```python
from build123d import *

# Parameters (mm, degrees)
SKETCH2_R           = 2.5
BOSS_EXTRUDE1_DEPTH = 5
SKETCH3_R           = 2.5
SKETCH3_R_2         = 0.5
BOSS_EXTRUDE2_DEPTH = 15.4


with BuildPart() as part:
    # Sketch2 → Boss-Extrude1 (new body)
    with BuildSketch(Plane.XY):
        with BuildLine():
            Line((-62, 4), (0, 4))
            ThreePointArc((0, 4), (1.530733729, 3.69551813), (2.828427125, 2.828427125))
            Line((2.828427125, 2.828427125), (17.67766953, -12.02081528))
            ThreePointArc((17.67766953, -12.02081528), (18.382077171, -16.725163117), (14.09037667, -18.776598105))
            Line((14.09037667, -18.776598105), (-62.758865735, -3.9273557))
            ThreePointArc((-62.758865735, -3.9273557), (-65.981797509, 0.381167417), (-62, 4))
        make_face()
        with Locations((-62, 0)):
            Circle(SKETCH2_R, mode=Mode.SUBTRACT)
        Circle(SKETCH2_R, mode=Mode.SUBTRACT)
    extrude(amount=BOSS_EXTRUDE1_DEPTH)

    # Sketch3 → Boss-Extrude2 (add)
    with BuildSketch(Plane(origin=(0, 0, 0), x_dir=(-1, 0, 0), z_dir=(0, 0, -1))):
        with Locations(Location((-14.849242405, -14.849242405, 0), (0, 0, 180))):
            Circle(SKETCH3_R)
        with Locations((-14.849242405, -14.849242405)):
            Circle(SKETCH3_R_2, mode=Mode.SUBTRACT)
    extrude(amount=BOSS_EXTRUDE2_DEPTH)


solid = part.part
```
Here's how the part is built. I have some questions about the finished solid (model axes, mm). A direction names the side the tool comes from. Coordinates: 2 decimals unless noted, no trailing zeros. Order: outer loops, then holes, each group sorted by start corner. A loop starts at its lowest first (then second) coordinate and runs counter-clockwise, first axis right, second up.
Item 1: If we section it at B-B, the plane y = -13.25: List the corners of the cut face in (x, z) for me, then the cut area to 3 significant figures.
Response values:
outline: (-14.51, 0) - (12.93, 0) - (12.93, -15.4) - (16.77, -15.4) - (16.77, 0) - (18.52, 0) - (18.52, 5) - (-14.51, 5) - close
area: 224 mm2
Item 2: I'm going to push flat-ended pins straight in: pin 1 Ø1.5 at (x, z) = (8, 1) entering from +Y; pin 2 Ø8 at (x, y) = (-23, -3) entering from -Z; pin 3 Ø4.5 at (x, y) = (-62, 0) entering from +Z; pin 4 Ø12 at (y, z) = (-7.5, -9.5) entering from +X. Where does each tip first touch, or does it pass through?
Response values:
pin 1: stops at y = -1.59
pin 2: stops at z = 0
pin 3: passes through
pin 4: stops at x = 16.95
Item 3: If we section it at C-C, the plane z = -6.5: List the corners of the cut face in (x, y) for me.
Response values:
outline: circle Ø5 at (14.85, -14.85); hole circle Ø1 at (14.85, -14.85)
Item 4: If we section it at A-A, the plane y = 1.5: List the corners of the cut face in (x, z) for me, then the cut area to 3 significant figures.
Response values:
outline: (-65.71, 0) - (-64, 0) - (-64, 5) - (-65.71, 5) - close; (-60, 0) - (-2, 0) - (-2, 5) - (-60, 5) - close; (2, 0) - (4.16, 0) - (4.16, 5) - (2, 5) - close
area: 309 mm2
Item 5: If we section it at D-D, the plane x = -38: List the corners of the cut face in (y, z) for me.
Response values:
outline: (-8.71, 0) - (4, 0) - (4, 5) - (-8.71, 5) - close
Item 6: Thinking about a two-plate mould opening in X: for faces 3 (the face through (-0.54, -2.44, 2.46)), 4 (the face through (-66, 0, 2)), 5 (the face through (-59.69, -0.96, 2.46)), 6 (the face through (-14, -5, 5)), which applies, pulls with the +X half, pulls with the -X half, needs draft (parallel to the pull), parting line crosses it, or undercut?
Response values:
face 3: undercut
face 4: pulls with the -X half
face 5: undercut
face 6: needs draft
Item 7: Which directions (+Z, -Z, +X, -X, +Y, -Y) give clear straight access to the entire face, cutting with the end or side of a thin tool? Please do faces 1 (the face through (16, -12.63, -7.59)), 2 (the face through (-31, 4, 2)).
Response values:
face 1: -Z
face 2: +Z, -Z, +X, -X, +Y
Item 8: I need wall thicknesses on probe 1 along Z at (x, y) = (-15.5, -0.5); probe 2 along X at (y, z) = (-14.5, -12.25); probe 3 along Y at (x, z) = (-62, 1.9). Which ranges of each line are inside material? Lowest first, please.
Response values:
probe 1: z = 0 to 5
probe 2: x = 12.37 to 14.49, 15.21 to 17.32
probe 3: y = -4.07 to -2.5, 2.5 to 4
